from build123d import *

# Parameters (mm, degrees)
BOSS_EXTRUDE1_DEPTH   = 1.5875
SKETCH3_R             = 4.445
SKETCH3_W             = 12.065
SKETCH3_H             = 12.065
CUT_EXTRUDE1_DEPTH    = 2.5875
SKETCH4_R             = 3.96875
CUT_EXTRUDE2_DEPTH    = 2.5875
SKETCH5_W             = 11.94
SKETCH5_H             = 20.64
SKETCH5_W_2           = 45.462
SKETCH5_H_2           = 102.32
SKETCH5_W_3           = 57
SKETCH5_H_3           = 15.1
CUT_EXTRUDE3_DEPTH    = 2.5875
SKETCH6_R             = 5.715
SKETCH6_W             = 14.605
SKETCH6_H             = 14.605
CUT_EXTRUDE4_DEPTH    = 2.5875
SKETCH7_W             = 66.04
SKETCH7_H             = 28.64
CUT_EXTRUDE5_DEPTH    = 2.5875
F_6_CLEARANCE_HOLE2_D = 4.3053
CUT_EXTRUDE6_START    = -1.5875
SKETCH12_W            = 13.529020254
SKETCH12_H            = 14.424558238
SKETCH12_W_2          = 13.332833864
SKETCH12_H_2          = 14.312726797
CUT_EXTRUDE6_DEPTH    = 1.5875


with BuildPart() as part:
    # Sketch1 → Boss-Extrude1 (new body)
    with BuildSketch(Plane.XY):
        with BuildLine():
            Line((74.93, -171.1167297), (86.51875, -171.1167297))
            Line((86.51875, -171.1167297), (86.51875, -67.9292297))
            Line((86.51875, -67.9292297), (-86.51875, -67.9292297))
            Line((-86.51875, -67.9292297), (-86.51875, -171.1167297))
            Line((-86.51875, -171.1167297), (-74.93, -171.1167297))
            ThreePointArc((-74.93, -171.1167297), (-71.337897552, -172.604627251), (-69.85, -176.1967297))
            Line((-69.85, -176.1967297), (-69.85, -182.2292297))
            Line((-69.85, -182.2292297), (69.85, -182.2292297))
            Line((69.85, -182.2292297), (69.85, -176.1967297))
            ThreePointArc((69.85, -176.1967297), (71.337897552, -172.604627251), (74.93, -171.1167297))
        make_face()
    extrude(amount=-BOSS_EXTRUDE1_DEPTH)

    # Sketch3 → Cut-Extrude1 (cut, through all)
    with BuildSketch(Plane.XY):
        with Locations((74.93, -159.3692297)):
            Circle(SKETCH3_R)
        with Locations((-6.731, -165.7192297)):
            Circle(SKETCH3_R)
        with Locations((-6.731, -145.3992297)):
            Circle(SKETCH3_R)
        with Locations((-6.731, -125.0792297)):
            Circle(SKETCH3_R)
        with Locations((-6.731, -104.7592297)):
            Circle(SKETCH3_R)
        with Locations((-6.731, -84.4392297)):
            Circle(SKETCH3_R)
        with Locations((-73.66, -139.0492297)):
            Rectangle(SKETCH3_W, SKETCH3_H)
        with Locations((13.843, -143.3672297)):
            Rectangle(SKETCH3_W, SKETCH3_H)
        with Locations((32.639, -143.3672297)):
            Rectangle(SKETCH3_W, SKETCH3_H)
        with Locations((51.435, -143.3672297)):
            Rectangle(SKETCH3_W, SKETCH3_H)
        with Locations((51.435, -124.5712297)):
            Rectangle(SKETCH3_W, SKETCH3_H)
        with Locations((32.639, -124.5712297)):
            Rectangle(SKETCH3_W, SKETCH3_H)
        with Locations((13.843, -124.5712297)):
            Rectangle(SKETCH3_W, SKETCH3_H)
        with Locations((13.843, -105.7752297)):
            Rectangle(SKETCH3_W, SKETCH3_H)
        with Locations((13.843, -86.9792297)):
            Rectangle(SKETCH3_W, SKETCH3_H)
        with Locations((32.639, -86.9792297)):
            Rectangle(SKETCH3_W, SKETCH3_H)
        with Locations((32.639, -105.7752297)):
            Rectangle(SKETCH3_W, SKETCH3_H)
        with Locations((51.435, -105.7752297)):
            Rectangle(SKETCH3_W, SKETCH3_H)
        with Locations((51.435, -86.9792297)):
            Rectangle(SKETCH3_W, SKETCH3_H)
    extrude(amount=-CUT_EXTRUDE1_DEPTH, mode=Mode.SUBTRACT)

    # Sketch4 → Cut-Extrude2 (cut, through all)
    with BuildSketch(Plane.XY):
        with Locations((-73.025, -113.9667297)):
            Circle(SKETCH4_R)
        with Locations((-73.025, -159.0517297)):
            Circle(SKETCH4_R)
        with Locations((74.295, -113.9667297)):
            Circle(SKETCH4_R)
        with Locations((75.184, -139.0492297)):
            Circle(SKETCH4_R)
    extrude(amount=-CUT_EXTRUDE2_DEPTH, mode=Mode.SUBTRACT)

    # Sketch5 → Cut-Extrude3 (cut, through all)
    with BuildSketch(Plane.XY):
        with Locations((-73.66, -84.3122297)):
            Rectangle(SKETCH5_W, SKETCH5_H)
        with Locations((73.66, -84.3122297)):
            Rectangle(SKETCH5_W, SKETCH5_H)
        with Locations((-39.799, -124.9522297)):
            Rectangle(SKETCH5_W_2, SKETCH5_H_2)
        with Locations((33.02, -165.4922297)):
            Rectangle(SKETCH5_W_3, SKETCH5_H_3)
    extrude(amount=-CUT_EXTRUDE3_DEPTH, mode=Mode.SUBTRACT)

    # Sketch6 → Cut-Extrude4 (cut, through all)
    with BuildSketch(Plane.XY):
        with Locations((74.93, -159.3692297)):
            Circle(SKETCH6_R)
        with Locations((-6.731, -165.7192297)):
            Circle(SKETCH6_R)
        with Locations((-6.731, -145.3992297)):
            Circle(SKETCH6_R)
        with Locations((-6.731, -125.0792297)):
            Circle(SKETCH6_R)
        with Locations((-6.731, -104.7592297)):
            Circle(SKETCH6_R)
        with Locations((-6.731, -84.4392297)):
            Circle(SKETCH6_R)
        with Locations((51.435, -143.3672297)):
            Rectangle(SKETCH6_W, SKETCH6_H)
        with Locations((51.435, -124.5712297)):
            Rectangle(SKETCH6_W, SKETCH6_H)
        with Locations((51.435, -105.7752297)):
            Rectangle(SKETCH6_W, SKETCH6_H)
        with Locations((51.435, -86.9792297)):
            Rectangle(SKETCH6_W, SKETCH6_H)
        with Locations((32.639, -143.3672297)):
            Rectangle(SKETCH6_W, SKETCH6_H)
        with Locations((32.639, -124.5712297)):
            Rectangle(SKETCH6_W, SKETCH6_H)
        with Locations((32.639, -105.7752297)):
            Rectangle(SKETCH6_W, SKETCH6_H)
        with Locations((32.639, -86.9792297)):
            Rectangle(SKETCH6_W, SKETCH6_H)
        with Locations((13.843, -86.9792297)):
            Rectangle(SKETCH6_W, SKETCH6_H)
        with Locations((13.843, -105.7752297)):
            Rectangle(SKETCH6_W, SKETCH6_H)
        with Locations((13.843, -124.5712297)):
            Rectangle(SKETCH6_W, SKETCH6_H)
        with Locations((13.843, -143.3672297)):
            Rectangle(SKETCH6_W, SKETCH6_H)
        with Locations((-73.66, -139.0492297)):
            Rectangle(SKETCH6_W, SKETCH6_H)
    extrude(amount=-CUT_EXTRUDE4_DEPTH, mode=Mode.SUBTRACT)

    # Sketch7 → Cut-Extrude5 (cut, through all)
    with BuildSketch(Plane.XY):
        with Locations((33.02, -162.5922297)):
            Rectangle(SKETCH7_W, SKETCH7_H)
    extrude(amount=-CUT_EXTRUDE5_DEPTH, mode=Mode.SUBTRACT)

    # #6 Clearance Hole2 (through all)
    with Locations(Plane(origin=(0, 0, 1.5875), x_dir=(-1, 0, 0), z_dir=(0, 0, 1))):
        with Locations((-81.28, 124.6982297), (6.731, 175.8792297), (81.28, 124.6982297), (6.731, 74.2792297)):
            Hole(F_6_CLEARANCE_HOLE2_D / 2)

    # Sketch12 → Cut-Extrude6 (cut)
    with BuildSketch(Plane(origin=(0, 0, -1.5875), x_dir=(-1, 0, 0), z_dir=(0, 0, -1)).offset(CUT_EXTRUDE6_START)):
        with Locations((73.612537257, -84.279184845)):
            Rectangle(SKETCH12_W, SKETCH12_H)
        with Locations((-73.648214967, -84.336507402)):
            Rectangle(SKETCH12_W_2, SKETCH12_H_2)
    extrude(amount=CUT_EXTRUDE6_DEPTH, mode=Mode.SUBTRACT)


solid = part.part
The model under review builds one solid part; all positions refer to its coordinate system, in mm. Give positions to 0.01 mm unless a question says otherwise; leave off trailing zeros. Loops run counter-clockwise (first coordinate to the right, second up) from the corner with the lowest first, then second, coordinate; pieces in that order, holes last. Notation, with made-up numbers: (-15.75, 0) -> (-8.75, 0) arc R13 cw to (-8.75, 15) -> close; hole circle Ø2 at (9, -35.75). An arc over 180 degrees is marked (long way). Write each question's results on one line, items separated by ' | '.
1) Draft analysis for pull direction X (two halves, no side actions). For faces 1 (the face through (6, -121, -1.588)), 2 (the face through (71.299, -172.644, -0.783)), 3 (the face through (-71.378, -172.565, -0.783)), 4 (the face through (74.324, -142.924, -0.783)), state which applies: pulls with the +X half, pulls with the -X half, needs draft (parallel to the pull), parting line crosses it, or undercut.
Conclusion:
face 1: needs draft | face 2: pulls with the +X half | face 3: pulls with the -X half | face 4: undercut
2) Take a section at A-A, the plane x = -59.5. Give the boundary of the cut face in (y, z).
Conclusion:
outline: (-182.23, -1.59) -> (-176.11, -1.59) -> (-176.11, 0) -> (-182.23, 0) -> close; (-73.79, -1.59) -> (-67.93, -1.59) -> (-67.93, 0) -> (-73.79, 0) -> close
3) Insertion check: pin 1 Ø15 at (x, y) = (-6.73, -165.72) entering from +Z; pin 2 Ø0.6 at (x, z) = (-80, -0.5) entering from -Y. Each pin has a flat end and moves straight along its axis. Give the tip position at first contact, or say it passes through.
Conclusion:
pin 1: stops at z = 0 | pin 2: stops at y = -171.12
4) Take a section at B-B, the plane y = -169. Give the boundary of the cut face in (x, z), plus the area to 3 significant figures.
Conclusion:
outline: (-86.52, -1.59) -> (-62.53, -1.59) -> (-62.53, 0) -> (-86.52, 0) -> close; (-17.07, -1.59) -> (-11.41, -1.59) -> (-11.41, 0) -> (-17.07, 0) -> close; (-2.05, -1.59) -> (0, -1.59) -> (0, 0) -> (-2.05, 0) -> close; (66.04, -1.59) -> (86.52, -1.59) -> (86.52, 0) -> (66.04, 0) -> close | area: 82.8 mm^2
5) For line 1 along X through (y, z) = (-135, -0.2); line 2 along Y through (x, z) = (26, -0.55); line 3 along Y through (x, z) = (-81.28, -0.75), list the stretches that pass through material, from the lowest coordinate up. Write a range as from..to.
Conclusion:
line 1: x = -86.52..-80.96, -66.36..-62.53, -17.07..86.52 | line 2: y = -182.23..-176.91, -136.06..-131.87, -117.27..-113.08, -98.47..-94.28, -79.68..-67.93 | line 3: y = -171.12..-126.85, -122.55..-67.93
6) Take a section at C-C, the plane z = -0.95. Count the separate pieces of the cut face and the enclosed holes in it, plus the area to 3 significant figures.
Conclusion:
separate pieces: 1 | enclosed holes: 28 | area: 8,800 mm^2
